```python
from build123d import *

# Parameters (mm, degrees)
BOSS_EXTRUDE1_DEPTH = 8
SKETCH2_R           = 2.5
CUT_EXTRUDE1_DEPTH  = 10
SKETCH3_R           = 2
CUT_EXTRUDE2_DEPTH  = 8
SKETCH4_R           = 2.5
CUT_EXTRUDE3_DEPTH  = 10
SKETCH5_R           = 2.5
CUT_EXTRUDE4_DEPTH  = 10
SKETCH6_R           = 3.5
CUT_EXTRUDE5_DEPTH  = 8


with BuildPart() as part:
    # Sketch1 → Boss-Extrude1 (new body)
    with BuildSketch(Plane.XY):
        Polygon((0, 38.2), (0, 22.2), (2, 22.2), (2, 0), (42, 0), (42, 174.5), (0, 174.5), (0, 166.2), (2, 166.2), (2, 146.2), (0, 146.2), (0, 130.2), (2, 130.2), (2, 110.2), (0, 110.2), (0, 94.2), (2, 94.2), (2, 74.2), (0, 74.2), (0, 58.2), (2, 58.2), (2, 38.2), align=None)
        Polygon((42, 174.5), (42, 0), (82, 0), (82, 22.2), (84, 22.2), (84, 38.2), (82, 38.2), (82, 58.2), (84, 58.2), (84, 74.2), (82, 74.2), (82, 94.2), (84, 94.2), (84, 110.2), (82, 110.2), (82, 130.2), (84, 130.2), (84, 146.2), (82, 146.2), (82, 166.2), (84, 166.2), (84, 174.5), align=None)
    extrude(amount=BOSS_EXTRUDE1_DEPTH)

    # Sketch2 → Cut-Extrude1 (cut)
    with BuildSketch(Plane.ZY.offset(-2)):
        with Locations(Location((4, 156.2, 0), (0, 0, 270))):
            Circle(SKETCH2_R)
        with Locations(Location((4, 120.2, 0), (0, 0, 270))):
            Circle(SKETCH2_R)
        with Locations(Location((4, 84.2, 0), (0, 0, 270))):
            Circle(SKETCH2_R)
        with Locations(Location((4, 48.2, 0), (0, 0, 270))):
            Circle(SKETCH2_R)
        with Locations(Location((4, 12.2, 0), (0, 0, 270))):
            Circle(SKETCH2_R)
    cut_extrude1 = extrude(amount=-CUT_EXTRUDE1_DEPTH, mode=Mode.SUBTRACT)

    # Mirror1: Cut-Extrude1 across plane
    add(cut_extrude1.mirror(Plane(origin=(42, 0, 0), x_dir=(0, 0, 1), z_dir=(1, 0, 0))), mode=Mode.SUBTRACT)

    # Sketch3 → Cut-Extrude2 (cut)
    with BuildSketch(Plane.XZ):
        with Locations(Location((42, 4, 0), (0, 0, 270))):
            Circle(SKETCH3_R)
        with Locations(Location((76, 4, 0), (0, 0, 270))):
            Circle(SKETCH3_R)
        with Locations(Location((8, 4, 0), (0, 0, 90))):
            Circle(SKETCH3_R)
    extrude(amount=-CUT_EXTRUDE2_DEPTH, mode=Mode.SUBTRACT)

    # Sketch4 → Cut-Extrude3 (cut)
    with BuildSketch(Plane(origin=(0, 174.5, 0), x_dir=(1, 0, 0), z_dir=(0, 1, 0))):
        with Locations(Location((5.75, -4, 0), (0, 0, 270))):
            Circle(SKETCH4_R)
        with Locations(Location((78.25, -4, 0), (0, 0, 90))):
            Circle(SKETCH4_R)
    extrude(amount=-CUT_EXTRUDE3_DEPTH, mode=Mode.SUBTRACT)

    # Sketch5 → Cut-Extrude4 (cut)
    with BuildSketch(Plane(origin=(0, 174.5, 0), x_dir=(1, 0, 0), z_dir=(0, 1, 0))):
        with Locations(Location((15.25, -4, 0), (0, 0, 270))):
            Circle(SKETCH5_R)
        with Locations(Location((31.25, -4, 0), (0, 0, 270))):
            Circle(SKETCH5_R)
    extrude(amount=-CUT_EXTRUDE4_DEPTH, mode=Mode.SUBTRACT)

    # Sketch6 → Cut-Extrude5 (cut)
    with BuildSketch(Plane.XY.offset(8)):
        with Locations((23, 161)):
            Circle(SKETCH6_R)
        with Locations(Location((61, 161, 0), (0, 0, 180))):
            Circle(SKETCH6_R)
    extrude(amount=-CUT_EXTRUDE5_DEPTH, mode=Mode.SUBTRACT)


solid = part.part
```
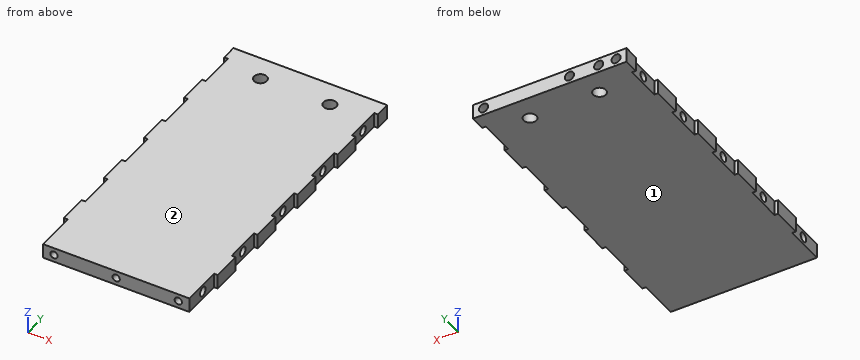
Design review of the part built by this model. Coordinates are the model's own, in mm. Face numbers are marked on the shaded views. Give positions to 0.01 mm unless a question says otherwise; leave off trailing zeros. Order: outer loops, then holes, each group sorted by start corner. A loop starts at its lowest first (then second) coordinate and runs counter-clockwise, first axis right, second up. Notation, with made-up numbers: (23, 19) -> (52, 19) arc R11 cw to (52, 31) -> close; hole circle Ø2 at (68, 8.5). An arc over 180 degrees is marked (long way). Write item = value, one per line. Start each with the question number.
(1) We need section D-D on x = 15.25. Write out the cut boundary in (y, z), plus the area to 3 significant figures.
(2) For pin 1 (1.6 mm diameter, centred on x = 83.5, z = 3.5, fed in from -Y); pin 2 (2 mm diameter, centred on x = 53, y = 115.5, fed in from -Z); pin 3 (4 mm diameter, centred on x = 78.25, z = 4, fed in from +Y); pin 4 (2.5 mm diameter, centred on y = 79, z = 2.5, fed in from +X), all flat-tipped, find the tip position at first contact; note any pin that passes through.
(3) We need section A-A on x = 61. Write out the cut boundary in (y, z).
(4) Mouldability with a two-part tool opening along Z and no side actions: class the marked faces 1 and 2 as +Z half, -Z half, draft (parallel to the pull), parting line (faces both ways), or undercut.
(5) To check wall thickness, follow line 1 along X through (y, z) = (168.5, 4); line 2 along Z through (x, y) = (78, 84); line 3 along Y through (x, z) = (23.5, 6). State the ranges of each line that lie inside material, in increasing order.
(6) We need section C-C on z = 4. State how many separate pieces and enclosed holes the cut face has, plus the area to 3 significant figures.
(7) We need section B-B on y = 84.2. Write out the cut boundary in (x, z).
Numbers:
q1.outline = (0, 0) -> (174.5, 0) -> (174.5, 1.5) -> (164.5, 1.5) -> (164.5, 6.5) -> (174.5, 6.5) -> (174.5, 8) -> (0, 8) -> close
q1.area = 1,350 mm^2
q2.pin_1 = 22.2
q2.pin_2 = 0
q2.pin_3 = 164.5
q2.pin_4 = 82
q3.outline = (0, 0) -> (157.5, 0) -> (157.5, 8) -> (0, 8) -> close; (164.5, 0) -> (174.5, 0) -> (174.5, 8) -> (164.5, 8) -> close
q4.face_1 = -Z half
q4.face_2 = +Z half
q5.line_1 = 0 to 3.25, 8.25 to 12.75, 17.75 to 28.75, 33.75 to 75.75, 80.75 to 84
q5.line_2 = 0 to 1.51, 6.49 to 8
q5.line_3 = 0 to 157.54, 164.46 to 174.5
q6.separate_pieces = 1
q6.enclosed_holes = 2
q6.area = 13,400 mm^2
q7.outline = (2, 0) -> (82, 0) -> (82, 1.5) -> (72, 1.5) -> (72, 6.5) -> (82, 6.5) -> (82, 8) -> (2, 8) -> (2, 6.5) -> (12, 6.5) -> (12, 1.5) -> (2, 1.5) -> close
